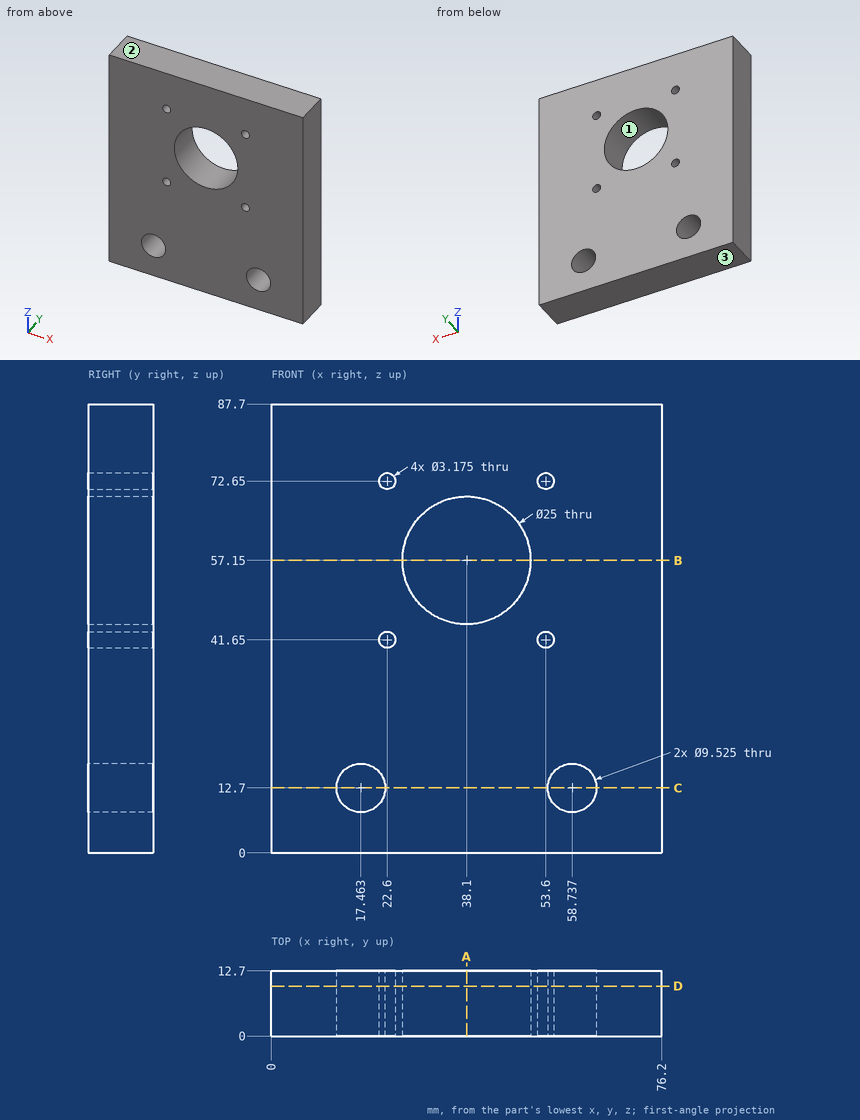
Part print with two shaded views. Sizes in mm from the minimum x, y, z corner. Coordinates: 2 decimals unless noted, no trailing zeros. Write each loop counter-clockwise with the first axis right and the second up, starting at its lowest first coordinate (ties: lowest second). Pieces come first, ordered by that corner, then holes.
(1) Cut at B-B on z = 57.15. List the corners of the cut face in (x, y), and give its area (3 significant figures).
(2) Pin check, flat tip, straight feed: pin 1 Ø1.9 at (x, z) = (53.6, 72.65) entering from +Y. Stop position of the tip, or through.
(3) Mould opens along Z. For the marked faces 1, 2 and 3 say: pulls with the +Z half, pulls with the -Z half, needs draft (parallel to the pull), parting line crosses it, or undercut.
(4) Cut at A-A on x = 38.1. List the corners of the cut face in (y, z), and give its area (3 significant figures).
(5) Cut at C-C on z = 12.7. List the corners of the cut face in (x, y) (1 decimal).
(6) Cut at D-D on y = 9.75. State how many separate pieces and enclosed holes the cut face has, and give its area (3 significant figures).
(7) Drill centre lines: line 1 (X direction, y = 8, z = 72.65); line 2 (Z direction, x = 22.6, y = 8.25); line 3 (Z direction, x = 58.5, y = 10.25). Where is each one in solid material? Low to high.
Working result:
1. outline: (0, 0) - (25.6, 0) - (25.6, 12.7) - (0, 12.7) - close; (50.6, 0) - (76.2, 0) - (76.2, 12.7) - (50.6, 12.7) - close
1. area: 650 mm2
2. pin 1: passes through
3. face 1: undercut
3. face 2: pulls with the +Z half
3. face 3: pulls with the -Z half
4. outline: (0, 0) - (12.7, 0) - (12.7, 44.65) - (0, 44.65) - close; (0, 69.65) - (12.7, 69.65) - (12.7, 87.7) - (0, 87.7) - close
4. area: 796 mm2
5. outline: (0, 0) - (12.7, 0) - (12.7, 12.7) - (0, 12.7) - close; (22.2, 0) - (54, 0) - (54, 12.7) - (22.2, 12.7) - close; (63.5, 0) - (76.2, 0) - (76.2, 12.7) - (63.5, 12.7) - close
6. separate pieces: 1
6. enclosed holes: 7
6. area: 6,020 mm2
7. line 1: x = 0 to 21.01, 24.19 to 52.01, 55.19 to 76.2
7. line 2: z = 0 to 40.06, 43.24 to 71.06, 74.24 to 87.7
7. line 3: z = 0 to 7.94, 17.46 to 87.7
